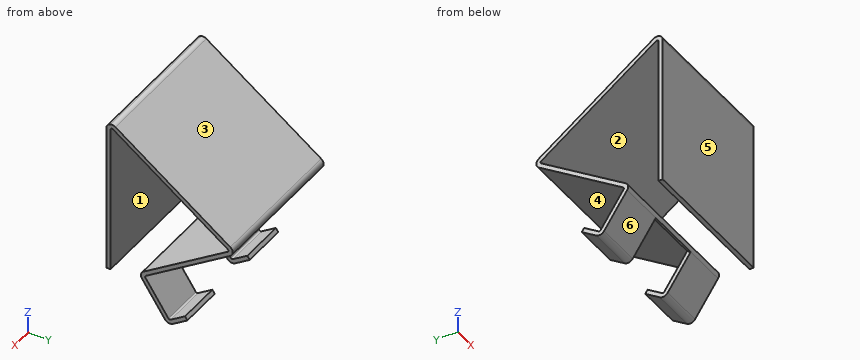
```python
from build123d import *

# Parameters (mm, degrees)
SKETCH1_W                      = 67.895404789
SKETCH1_H                      = 2
BASE_FLANGE1_DEPTH             = 37.5
EDGE_FLANGE1_START             = -28.961034246
EDGE_FLANGE1_DEPTH             = 67.895404789
EDGE_FLANGE1_2_DEPTH           = 67.895404789
EDGE_FLANGE2_START             = -28.961034246
EDGE_FLANGE2_DEPTH             = 67.895404789
EDGE_FLANGE2_2_DEPTH           = 67.895404789
EDGE_FLANGE3_STRIP_W           = 9.4732
EDGE_FLANGE3_STRIP_H           = 2
EDGE_FLANGE3_STRIP_CUT_DEPTH   = 67.89540479
EDGE_FLANGE3_DEPTH             = 67.89540479
CUT_EXTRUDE1_REACH             = 92.8
SKETCH15_W                     = 26.092581692
SKETCH15_H                     = 22.2634
EDGE_FLANGE4_STRIP_W           = 9.4732
EDGE_FLANGE4_STRIP_H           = 2
EDGE_FLANGE4_STRIP_CUT_DEPTH   = 20.44630838
EDGE_FLANGE4_STRIP_2_W         = 9.4732
EDGE_FLANGE4_STRIP_2_H         = 2
EDGE_FLANGE4_STRIP_CUT_2_DEPTH = 21.356514718
EDGE_FLANGE4_DEPTH             = 20.44630838
EDGE_FLANGE4_BEND_DEPTH        = 21.356514718


# Read off the part's stored shape, not the designer's step: Edge-Flange1, Edge-Flange2
# Sheet-metal steps are written as plain solids
with BuildPart() as part:
    # Sketch1 → Base-Flange1 (new, symmetric)
    with BuildSketch(Plane.XY):
        with Locations((4.986668148, 1)):
            Rectangle(SKETCH1_W, SKETCH1_H)
    extrude(amount=BASE_FLANGE1_DEPTH, both=True)

    # Edge-Flange1 outline → Edge-Flange1 (cut)
    with BuildSketch(Plane.YZ.offset(EDGE_FLANGE1_START)):
        with BuildLine():
            ThreePointArc((0, 33.643455388), (0.556604688, 35.297722597), (2, 36.279057786))
            Line((2, 36.279057786), (2, 37.5))
            Line((2, 37.5), (0, 37.5))
            Line((0, 37.5), (0, 33.643455388))
        make_face()
    extrude(amount=EDGE_FLANGE1_DEPTH, mode=Mode.SUBTRACT)

    # Edge-Flange1 2 outline → Edge-Flange1 2 (add)
    with BuildSketch(Plane.YZ.offset(EDGE_FLANGE1_START)):
        with BuildLine():
            Line((61.436403322, -4.11781765), (4.306249276, 35.885146872))
            ThreePointArc((4.306249276, 35.885146872), (3.197343124, 36.340990436), (2, 36.279057786))
            Line((2, 36.279057786), (2, 33.643455388))
            ThreePointArc((2, 33.643455388), (2.396475972, 34.296827567), (3.159096403, 34.246842784))
            Line((3.159096403, 34.246842784), (60.289250449, -5.756121738))
            Line((60.289250449, -5.756121738), (61.436403322, -4.11781765))
        make_face()
    extrude(amount=EDGE_FLANGE1_2_DEPTH)

    # Edge-Flange2 outline → Edge-Flange2 (cut)
    with BuildSketch(Plane.YZ.offset(EDGE_FLANGE2_START)):
        with BuildLine():
            ThreePointArc((58.80360799, -2.274314512), (59.839449023, -3.679107071), (59.81541421, -5.424338031))
            Line((59.81541421, -5.424338031), (60.289250449, -5.756121738))
            Line((60.289250449, -5.756121738), (61.436403322, -4.11781765))
            Line((61.436403322, -4.11781765), (58.80360799, -2.274314512))
        make_face()
    extrude(amount=EDGE_FLANGE2_DEPTH, mode=Mode.SUBTRACT)

    # Edge-Flange2 2 outline → Edge-Flange2 2 (add)
    with BuildSketch(Plane.YZ.offset(EDGE_FLANGE2_START)):
        with BuildLine():
            Line((16.468222849, -35.313778071), (58.764246014, -6.784750218))
            ThreePointArc((58.764246014, -6.784750218), (59.399434997, -6.189234023), (59.81541421, -5.424338031))
            Line((59.81541421, -5.424338031), (57.656455118, -3.912618601))
            ThreePointArc((57.656455118, -3.912618601), (57.970530667, -4.522433963), (57.645860207, -5.126675073))
            Line((57.645860207, -5.126675073), (15.349837042, -33.655702926))
            Line((15.349837042, -33.655702926), (16.468222849, -35.313778071))
        make_face()
    extrude(amount=EDGE_FLANGE2_2_DEPTH)

    # Edge-Flange3 strip (across the edge) → Edge-Flange3 strip cut (cut)
    with BuildSketch(Plane(origin=(38.934370543, 16.468222849, -35.313778071), x_dir=(0, 0.829037572555041, 0.5591929034707481), z_dir=(-1, 0, 0))):
        with Locations((-2, -1)):
            Rectangle(EDGE_FLANGE3_STRIP_W, EDGE_FLANGE3_STRIP_H)
    extrude(amount=EDGE_FLANGE3_STRIP_CUT_DEPTH, mode=Mode.SUBTRACT)

    # Edge-Flange3 section (across the edge) → Edge-Flange3 (add)
    with BuildSketch(Plane(origin=(38.934370543, 16.468222849, -35.313778071), x_dir=(0, 0.829037572555041, 0.5591929034707481), z_dir=(-1, 0, 0))):
        with BuildLine():
            Line((0, 0.7366), (0, 23))
            Line((0, 23), (2, 23))
            Line((2, 23), (2, 0.7366))
            ThreePointArc((2, 0.7366), (2.215745145, 0.215745145), (2.7366, 0))
            Line((2.7366, 0), (2.7366, -2))
            ThreePointArc((2.7366, -2), (0.801531583, -1.198468417), (0, 0.7366))
        make_face()
    extrude(amount=EDGE_FLANGE3_DEPTH)

    # Sketch15 → Cut-Extrude1 (cut, up to next)
    with BuildSketch(Plane(origin=(0, -3.394443435, -2.289581007), x_dir=(1, 0, 0), z_dir=(0, 0.8290375725550408, 0.559192903470748)), mode=Mode.PRIVATE) as cut_extrude1_sk1:
        with Locations((5.441771317, 50.3536622)):
            Rectangle(SKETCH15_W, SKETCH15_H)
    cut_extrude1_tool1 = extrude(cut_extrude1_sk1.sketch, amount=-CUT_EXTRUDE1_REACH, mode=Mode.PRIVATE) & part.part
    add(cut_extrude1_tool1.solids().sort_by_distance((5.441771, 24.762967, -44.034659))[0], mode=Mode.SUBTRACT)

    # Edge-Flange4 strip (across the edge) → Edge-Flange4 strip cut (cut)
    with BuildSketch(Plane(origin=(38.934370543, 30.987734774, -53.263256433), x_dir=(0, -0.5591929034707451, 0.8290375725550428), z_dir=(-1, 0, 0))):
        with Locations((-2, -1)):
            Rectangle(EDGE_FLANGE4_STRIP_W, EDGE_FLANGE4_STRIP_H)
    extrude(amount=EDGE_FLANGE4_STRIP_CUT_DEPTH, mode=Mode.SUBTRACT)

    # Edge-Flange4 strip 2 (across the edge) → Edge-Flange4 strip cut 2 (cut)
    with BuildSketch(Plane(origin=(-7.604519529, 30.987734774, -53.263256433), x_dir=(0, -0.5591929034707451, 0.8290375725550428), z_dir=(-1, 0, 0))):
        with Locations((-2, -1)):
            Rectangle(EDGE_FLANGE4_STRIP_2_W, EDGE_FLANGE4_STRIP_2_H)
    extrude(amount=EDGE_FLANGE4_STRIP_CUT_2_DEPTH, mode=Mode.SUBTRACT)

    # Edge-Flange4 section (across the edge) → Edge-Flange4 (add)
    with BuildSketch(Plane(origin=(38.934370543, 30.987734774, -53.263256433), x_dir=(0, -0.5591929034707451, 0.8290375725550428), z_dir=(-1, 0, 0))):
        with BuildLine():
            Line((0, 0.7366), (0, 9))
            Line((0, 9), (2, 9))
            Line((2, 9), (2, 0.7366))
            ThreePointArc((2, 0.7366), (2.215745145, 0.215745145), (2.7366, 0))
            Line((2.7366, 0), (2.7366, -2))
            ThreePointArc((2.7366, -2), (0.801531583, -1.198468417), (0, 0.7366))
        make_face()
    extrude(amount=EDGE_FLANGE4_DEPTH)

    # Edge-Flange4 section 2 (across the edge) → Edge-Flange4 bend (add)
    with BuildSketch(Plane(origin=(-7.604519529, 30.987734774, -53.263256433), x_dir=(0, -0.5591929034707451, 0.8290375725550428), z_dir=(-1, 0, 0))):
        with BuildLine():
            Line((0, 0.7366), (0, 9))
            Line((0, 9), (2, 9))
            Line((2, 9), (2, 0.7366))
            ThreePointArc((2, 0.7366), (2.215745145, 0.215745145), (2.7366, 0))
            Line((2.7366, 0), (2.7366, -2))
            ThreePointArc((2.7366, -2), (0.801531583, -1.198468417), (0, 0.7366))
        make_face()
    extrude(amount=EDGE_FLANGE4_BEND_DEPTH)


solid = part.part
```
Input: part model. Units: mm. Frame: model coordinates. Face numbers are marked on the shaded views. A direction names the side the tool comes from. Give positions to 0.01 mm unless a question says otherwise; leave off trailing zeros. Loops run counter-clockwise (first coordinate to the right, second up) from the corner with the lowest first, then second, coordinate; pieces in that order, holes last.
1) Section query B-B on x = -21. Return the cut outline in (y, z).
A:
outline: (0, -37.5) - (2, -37.5) - (2, 33.64) arc R0.74 cw to (3.16, 34.25) - (57.66, -3.91) arc R0.74 cw to (57.65, -5.13) - (17.62, -32.13) arc R2.74 ccw to (16.88, -35.92) - (27.8, -52.11) arc R2.74 ccw to (31.6, -52.85) - (38.45, -48.23) - (37.33, -46.57) - (30.48, -51.19) arc R0.74 cw to (29.46, -50.99) - (18.54, -34.81) arc R0.74 cw to (18.74, -33.78) - (58.76, -6.78) arc R2.74 ccw to (58.8, -2.27) - (4.31, 35.89) arc R2.74 ccw to (0, 33.64) - close
2) Mould query, pull axis Z, two halves, no side actions, for the marked faces 3, 4, 5 and 6. Classes: released by +Z, released by -Z, zero draft, split by the parting line, or undercut.
A:
face 3: released by +Z
face 4: undercut
face 5: zero draft
face 6: released by -Z
3) Section query C-C on z = 27. Return the cut outline in (x, y), and give its area (3 significant figures).
A:
outline: (-28.96, 0) - (38.93, 0) - (38.93, 2) - (-28.96, 2) - close; (-28.96, 13.51) - (38.93, 13.51) - (38.93, 17) - (-28.96, 17) - close
area: 373 mm2
4) Section query D-D on x = 8.5. Return the cut outline in (y, z).
A:
outline: (0, -37.5) - (2, -37.5) - (2, 33.64) arc R0.74 cw to (3.16, 34.25) - (57.66, -3.91) arc R0.74 cw to (57.65, -5.13) - (17.62, -32.13) arc R2.74 ccw to (16.88, -35.92) - (18.54, -34.81) arc R0.74 cw to (18.74, -33.78) - (58.76, -6.78) arc R2.74 ccw to (58.8, -2.27) - (4.31, 35.89) arc R2.74 ccw to (0, 33.64) - close
5) Line query: L1, parallel to Z at x = -17, y = 20.5; L2, parallel to Z at x = 19, y = 26; L3, parallel to Z at x = 34, y = 40. Output: solid intervals per line, ascending.
A:
L1: z = -41.29 to -37.71, -32.59 to -30.18, 22.1 to 24.55
L2: z = -49.45 to -45.87, -28.88 to -26.47, 18.25 to 20.7
L3: z = -19.44 to -17.03, 8.45 to 10.89
6) Reachability of the marked faces 1 and 2 from +Z, -Z, +X, -X, +Y, -Y: full face, straight path, thin tool, end or side. Return the list, or none.
A:
face 1: -Z, +X, -X
face 2: +X, -X
7) Contact query for flat-ended pins moving along their axis: pin 1 (1.6 mm diameter, centred on x = 13, y = 0.5, fed in from -Z); pin 2 (6 mm diameter, centred on x = 1.5, y = 43.5, fed in from -Z); pin 3 (5 mm diameter, centred on x = 18, y = 34, fed in from -Z). Output: stop coordinate, or through.
A:
pin 1: stops at z = -37.5
pin 2: stops at z = -19.1
pin 3: stops at z = -52.88
8) Section query A-A on y = 44. Return the cut outline in (x, z).
A:
outline: (-28.96, -16.74) - (38.93, -16.74) - (38.93, -14.33) - (-28.96, -14.33) - close; (-28.96, 5.65) - (38.93, 5.65) - (38.93, 8.09) - (-28.96, 8.09) - close
